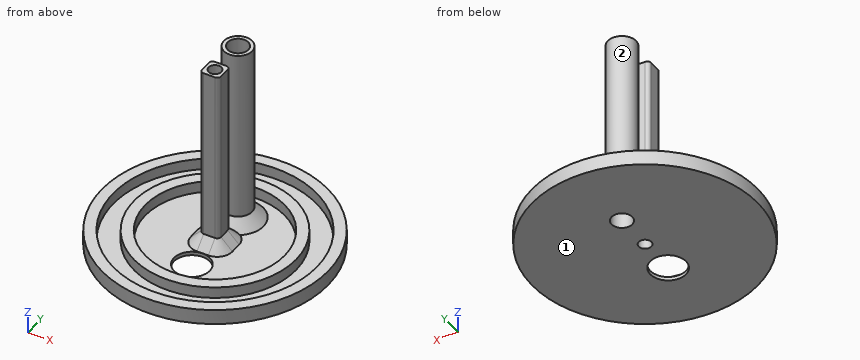
from build123d import *

# Parameters (mm, degrees)
F0_R         = 30
F0_R_2       = 27
F0_R_3       = 21.5
F0_R_4       = 18.5
F0_R_5       = 4.75
F0_W         = 5
F0_H         = 5
F0_R_6       = 3.75
F0_R_7       = 1.7
F1_DEPTH     = 1
F2_DEPTH     = 4
F0_R_8       = 2.75
F3_DEPTH     = 50
F4_R         = 1
F5_T1_DEPTH  = 3
F5_T3_DEPTH  = 3
F5_T6_ANGLE  = 90
F5_T10_ANGLE = 90
F5_T12_ANGLE = 90
F5_T14_ANGLE = 90


# Not quite as in the source:
# - a fillet or chamfer that OpenCascade refuses, or shapes differently, is made with other operations: its cross-section is extruded or revolved along the edge and cut away or added


with BuildPart() as f1:
    # F0 (on Top) → F1 (new body)
    with BuildSketch(Plane.XY):
        Circle(F0_R)
        Circle(F0_R_2, mode=Mode.SUBTRACT)
        Circle(F0_R_2)
        Circle(F0_R_3, mode=Mode.SUBTRACT)
        Circle(F0_R_3)
        Circle(F0_R_4, mode=Mode.SUBTRACT)
        Circle(F0_R_4)
        with Locations((0, -10.3181230716)):
            Circle(F0_R_5, mode=Mode.SUBTRACT)
        with Locations((0, -0.0181230716)):
            Rectangle(F0_W, F0_H, mode=Mode.SUBTRACT)
        with Locations((0, 10.2818769284)):
            Circle(F0_R_6, mode=Mode.SUBTRACT)
        with Locations((0, -0.0181230716)):
            Rectangle(F0_W, F0_H)
        with Locations((0, -0.0181230716)):
            Circle(F0_R_7, mode=Mode.SUBTRACT)
    extrude(amount=F1_DEPTH)

    # F0 (on Top) → F2 (join)
    with BuildSketch(Plane.XY):
        Circle(F0_R)
        Circle(F0_R_2, mode=Mode.SUBTRACT)
        Circle(F0_R_3)
        Circle(F0_R_4, mode=Mode.SUBTRACT)
    extrude(amount=F2_DEPTH)

    # F0 (on Top) → F3 (join)
    with BuildSketch(Plane.XY):
        with Locations((0, -0.0181230716)):
            Rectangle(F0_W, F0_H)
        with Locations((0, -0.0181230716)):
            Circle(F0_R_7, mode=Mode.SUBTRACT)
        with Locations((0, 10.2818769284)):
            Circle(F0_R_6)
        with Locations((0, 10.2818769284)):
            Circle(F0_R_8, mode=Mode.SUBTRACT)
    extrude(amount=F3_DEPTH)

    # F4
    f4_edges = [f1.edges().sort_by_distance(p)[0] for p in [
        (-2.5, -2.518123, 25.5),
        (2.5, -2.518123, 25.5),
        (-2.5, 2.481877, 25.5),
        (2.5, 2.481877, 25.5),
    ]]
    fillet(f4_edges, radius=F4_R)

    # F5: chamfer of 3 on 3 edges, made by hand

    # F5_s2 → F5_t1 (join)
    with BuildSketch(Plane.YZ.offset(-1.5)):
        Polygon((-5.5181230716, 1), (-2.5181230716, 4), (-2.5181230716, 1), align=None)
        Polygon((5.4818769284, 1), (2.4818769284, 4), (2.4818769284, 1), align=None)
    extrude(amount=F5_T1_DEPTH)

    # F5_s4 → F5_t3 (join)
    with BuildSketch(Plane.XZ.offset(-1.4818769284)):
        Polygon((-5.5, 1), (-2.5, 4), (-2.5, 1), align=None)
        Polygon((5.5, 1), (2.5, 4), (2.5, 1), align=None)
    extrude(amount=F5_T3_DEPTH)

    # F5_s5 → F5_t6 (revolve)
    with BuildSketch(Plane.YZ.offset(-1.5)):
        Polygon((-5.5181230716, 1), (-2.5181230716, 4), (-2.5181230716, 1), align=None)
    revolve(axis=Axis((-1.5, -1.5181230716, 1), (0, 0, -1)), revolution_arc=F5_T6_ANGLE)

    # F5_s7 → F5_t8 (revolve)
    with BuildSketch(Plane.XZ.offset(-10.2818769284)):
        Polygon((6.75, 1), (3.75, 4), (3.75, 1), align=None)
    revolve(axis=Axis((0, 10.2818769284, 1), (0, 0, 1)))

    # F5_s9 → F5_t10 (revolve)
    with BuildSketch(Plane.XZ.offset(-1.4818769284)):
        Polygon((-5.5, 1), (-2.5, 4), (-2.5, 1), align=None)
    revolve(axis=Axis((-1.5, 1.4818769284, 1), (0, 0, -1)), revolution_arc=F5_T10_ANGLE)

    # F5_s11 → F5_t12 (revolve)
    with BuildSketch(Plane.YZ.offset(1.5)):
        Polygon((5.4818769284, 1), (2.4818769284, 4), (2.4818769284, 1), align=None)
    revolve(axis=Axis((1.5, 1.4818769284, 1), (0, 0, -1)), revolution_arc=F5_T12_ANGLE)

    # F5_s13 → F5_t14 (revolve)
    with BuildSketch(Plane.YZ.offset(1.5)):
        Polygon((-5.5181230716, 1), (-2.5181230716, 4), (-2.5181230716, 1), align=None)
    revolve(axis=Axis((1.5, -1.5181230716, 1), (0, 0, 1)), revolution_arc=F5_T14_ANGLE)


solid = f1.part
Geometry check sheet. Reference: the model listing, model coordinates, mm. Face numbers are marked on the shaded views. Give positions to 0.01 mm unless a question says otherwise; leave off trailing zeros. Order: outer loops, then holes, each group sorted by start corner. A loop starts at its lowest first (then second) coordinate and runs counter-clockwise, first axis right, second up. Notation, with made-up numbers: (-1.75, -31.5) - (53.25, -31.5) arc R11 cw to (53.25, -26.5) - close; hole circle Ø11 at (-5, -23). An arc over 180 degrees is marked (long way). Answer as a JSON object with one key per item and string values.
(1) Cross-section at A-A (z = 20). Record the cut outline in (x, y).
Report:
{"outline": "circle Ø7.5 at (0, 10.28); (-2.5, -1.52) arc R1 ccw to (-1.5, -2.52) - (1.5, -2.52) arc R1 ccw to (2.5, -1.52) - (2.5, 1.48) arc R1 ccw to (1.5, 2.48) - (-1.5, 2.48) arc R1 ccw to (-2.5, 1.48) - close; hole circle Ø5.5 at (0, 10.28); hole circle Ø3.4 at (0, -0.02)"}
(2) Depth check by flat-ended pin: pin 1 Ø16 at (x, y) = (-13, 9) entering from +Z; pin 2 Ø1 at (x, y) = (-12, 12.5) entering from +Z; pin 3 Ø0.9 at (x, z) = (0, 16.5) entering from +Y. Enter the tip coordinate at first touch or a pass-through.
Report:
{"pin 1": "z = 4", "pin 2": "z = 1", "pin 3": "y = 14.03"}
(3) Cross-section at C-C (y = 23.5). Record the cut outline in (x, z), then the cut area to 3 significant figures.
Report:
{"outline": "(-18.65, 0) - (18.65, 0) - (18.65, 4) - (13.29, 4) - (13.29, 1) - (-13.29, 1) - (-13.29, 4) - (-18.65, 4) - close", "area": "69.4 mm^2"}
(4) Draft check along Y on the marked faces 1 and 2. Enter one of: released by +Y, released by -Y, zero draft, split by the parting line, or undercut.
Report:
{"face 1": "zero draft", "face 2": "undercut"}
(5) Cross-section at B-B (x = -17). Record the cut outline in (y, z).
Report:
{"outline": "(-24.72, 0) - (24.72, 0) - (24.72, 4) - (20.98, 4) - (20.98, 1) - (13.16, 1) - (13.16, 4) - (7.3, 4) - (7.3, 1) - (-7.3, 1) - (-7.3, 4) - (-13.16, 4) - (-13.16, 1) - (-20.98, 1) - (-20.98, 4) - (-24.72, 4) - close"}
(6) Material ranges on line 1 (Y direction, x = 0, z = 0.35); line 2 (Y direction, x = 0, z = 33); line 3 (X direction, y = 10, z = 27), recorded low to high.
Report:
{"line 1": "-30 to -15.07, -5.57 to -1.72, 1.68 to 7.53, 13.03 to 30", "line 2": "-2.52 to -1.72, 1.68 to 2.48, 6.53 to 7.53, 13.03 to 14.03", "line 3": "-3.74 to -2.74, 2.74 to 3.74"}
(7) Cross-section at D-D (x = 0). State how many separate pieces and enclosed holes the cut face has, then the cut area to 3 significant figures.
Report:
{"separate pieces": "4", "enclosed holes": "0", "area": "271 mm^2"}
